Geometry: final body of the model. Coordinates: model frame, mm. A direction names the side the tool comes from. Give positions to 0.01 mm unless a question says otherwise; leave off trailing zeros. Order: outer loops, then holes, each group sorted by start corner. A loop starts at its lowest first (then second) coordinate and runs counter-clockwise, first axis right, second up. Notation, with made-up numbers: (-3.5, 66.25) - (35.5, 66.25) arc R31 cw to (35.5, 90.25) - close; hole circle Ø8 at (10, 89.25). An arc over 180 degrees is marked (long way). Use one line per item in the form item = value.
from build123d import *

# Parameters (mm, degrees)
SKETCH1_W           = 117.5
SKETCH1_H           = 85
BOSS_EXTRUDE1_DEPTH = 3
SKETCH2_W           = 17.5
SKETCH2_H           = 5
BOSS_EXTRUDE2_DEPTH = 94
SKETCH3_W           = 17.5
SKETCH3_H           = 20
SKETCH3_R           = 2.1
BOSS_EXTRUDE3_DEPTH = 5
CHAMFER1_SIZE       = 2
CHAMFER2_SIZE       = 3
FILLET1_R           = 4.2


with BuildPart() as part:
    # Sketch1 → Boss-Extrude1 (new body)
    with BuildSketch(Plane(origin=(0, 0, 0), x_dir=(1, 0, 0), z_dir=(0, 1, 0))):
        Rectangle(SKETCH1_W, SKETCH1_H)
    extrude(amount=BOSS_EXTRUDE1_DEPTH)

    # Sketch2 → Boss-Extrude2 (add)
    with BuildSketch(Plane(origin=(0, 3, 0), x_dir=(1, 0, 0), z_dir=(0, 1, 0))):
        with Locations((-50, 40)):
            Rectangle(SKETCH2_W, SKETCH2_H)
        with Locations((50, 40)):
            Rectangle(SKETCH2_W, SKETCH2_H)
        with Locations((50, -40)):
            Rectangle(SKETCH2_W, SKETCH2_H)
        with Locations((-50, -40)):
            Rectangle(SKETCH2_W, SKETCH2_H)
    extrude(amount=BOSS_EXTRUDE2_DEPTH)

    # Sketch3 → Boss-Extrude3 (add)
    # profile 1 of 4: a face of its own
    with BuildSketch(Plane(origin=(0, 97, 0), x_dir=(1, 0, 0), z_dir=(0, 1, 0))):
        with Locations((-50, 47.5)):
            Rectangle(SKETCH3_W, SKETCH3_H)
        with Locations(Location((-50, 50, 0), (0, 0, 270))):
            Circle(SKETCH3_R, mode=Mode.SUBTRACT)
    # profile 2 of 4: a face of its own
    with BuildSketch(Plane(origin=(0, 97, 0), x_dir=(1, 0, 0), z_dir=(0, 1, 0))):
        with Locations((50, 47.5)):
            Rectangle(SKETCH3_W, SKETCH3_H)
        with Locations(Location((50, 50, 0), (0, 0, 90))):
            Circle(SKETCH3_R, mode=Mode.SUBTRACT)
    # profile 3 of 4: a face of its own
    with BuildSketch(Plane(origin=(0, 97, 0), x_dir=(1, 0, 0), z_dir=(0, 1, 0))):
        with Locations((50, -47.5)):
            Rectangle(SKETCH3_W, SKETCH3_H)
        with Locations(Location((50, -50, 0), (0, 0, 270))):
            Circle(SKETCH3_R, mode=Mode.SUBTRACT)
    # profile 4 of 4: a face of its own
    with BuildSketch(Plane(origin=(0, 97, 0), x_dir=(1, 0, 0), z_dir=(0, 1, 0))):
        with Locations((-50, -47.5)):
            Rectangle(SKETCH3_W, SKETCH3_H)
        with Locations(Location((-50, -50, 0), (0, 0, 90))):
            Circle(SKETCH3_R, mode=Mode.SUBTRACT)
    extrude(amount=-BOSS_EXTRUDE3_DEPTH)

    # Chamfer1
    chamfer1_edges = [part.edges().sort_by_distance(p)[0] for p in [
        (50, 92, 47.9),
        (-50, 92, 52.1),
        (-50, 92, -52.1),
        (50, 92, -47.9),
    ]]
    chamfer(chamfer1_edges, length=CHAMFER1_SIZE)

    # Chamfer2
    chamfer2_edges = [part.edges().sort_by_distance(p)[0] for p in [
        (50, 92, 42.5),
        (-50, 92, 42.5),
        (-50, 92, -42.5),
        (50, 92, -42.5),
    ]]
    chamfer(chamfer2_edges, length=CHAMFER2_SIZE)

    # Fillet1
    fillet1_edges = [part.edges().sort_by_distance(p)[0] for p in [
        (41.25, 94.5, 57.5),
        (58.75, 94.5, 57.5),
        (-58.75, 94.5, 57.5),
        (-41.25, 94.5, 57.5),
        (-41.25, 94.5, -57.5),
        (-58.75, 94.5, -57.5),
        (58.75, 94.5, -57.5),
        (41.25, 94.5, -57.5),
    ]]
    fillet(fillet1_edges, radius=FILLET1_R)


solid = part.part
(1) Cut plane D-D on z = -39.5. Output: boundary loops of the cut face in (x, y).
Computed values:
outline = (-58.75, 0) - (58.75, 0) - (58.75, 97) - (41.25, 97) - (41.25, 3) - (-41.25, 3) - (-41.25, 97) - (-58.75, 97) - close
(2) Cut plane C-C on z = 50. Output: boundary loops of the cut face in (x, y), plus the area to 3 significant figures.
Computed values:
outline = (-58.75, 92) - (-54.1, 92) - (-52.1, 94) - (-52.1, 97) - (-58.75, 97) - close; (-47.9, 94) - (-45.9, 92) - (-41.25, 92) - (-41.25, 97) - (-47.9, 97) - close; (41.25, 92) - (45.9, 92) - (47.9, 94) - (47.9, 97) - (41.25, 97) - close; (52.1, 94) - (54.1, 92) - (58.75, 92) - (58.75, 97) - (52.1, 97) - close
area = 125 mm²
(3) Cut plane B-B on x = -50. Output: boundary loops of the cut face in (y, z).
Computed values:
outline = (0, -42.5) - (89, -42.5) - (92, -45.5) - (92, -45.9) - (94, -47.9) - (97, -47.9) - (97, -37.5) - (3, -37.5) - (3, 37.5) - (97, 37.5) - (97, 47.9) - (94, 47.9) - (92, 45.9) - (92, 45.5) - (89, 42.5) - (0, 42.5) - close; (92, -57.5) - (97, -57.5) - (97, -52.1) - (94, -52.1) - (92, -54.1) - close; (92, 54.1) - (94, 52.1) - (97, 52.1) - (97, 57.5) - (92, 57.5) - close
(4) Ray query, line 1 along X through (y, z) = (95.7, 50); line 2 along Z through (x, y) = (-43, 45); line 3 along Y through (x, z) = (23.5, -32). Return the intervals inside material, ascending.
Computed values:
line_1 = -58.75 to -52.1, -47.9 to -41.25, 41.25 to 47.9, 52.1 to 58.75
line_2 = -42.5 to -37.5, 37.5 to 42.5
line_3 = 0 to 3
(5) Pull-direction query (X, two-part tool) for faces 1 (the face through (58.75, 41, 40)), 2 (the face through (-48.137, 95.521, 49.031)), 3 (the face through (50, 95, 57.5)), 4 (the face through (42.45, 94.46, 56.24)); classes: released by +X, released by -X, zero draft, split by the parting line, or undercut.
Computed values:
face_1 = released by +X
face_2 = undercut
face_3 = zero draft
face_4 = undercut
(6) Cut plane A-A on y = 24.5. Output: boundary loops of the cut face in (x, z).
Computed values:
outline = (-58.75, -42.5) - (-41.25, -42.5) - (-41.25, -37.5) - (-58.75, -37.5) - close; (-58.75, 37.5) - (-41.25, 37.5) - (-41.25, 42.5) - (-58.75, 42.5) - close; (41.25, -42.5) - (58.75, -42.5) - (58.75, -37.5) - (41.25, -37.5) - close; (41.25, 37.5) - (58.75, 37.5) - (58.75, 42.5) - (41.25, 42.5) - close
(7) Contact query for flat-ended pins moving along their axis: pin 1 Ø9.5 at (x, z) = (-46, 51.5) entering from -Y; pin 2 Ø3.5 at (x, z) = (-50, -50) entering from +Y; pin 3 Ø9.5 at (x, z) = (-51.5, -48.5) entering from -Y; pin 4 Ø5 at (x, y) = (-47, 65.5) entering from +Z. Output: stop coordinate, or through.
Computed values:
pin_1 = 92
pin_2 = through
pin_3 = 90.25
pin_4 = 42.5
(8) Reachability of faces 5 (the face through (4, 1, 42.5)), 6 (the face through (49.9, 97, -47.6)), 7 (the face through (-41.25, 53, -42)), 8 (the face through (-50, 49, -37.5)) from +Z, -Z, +X, -X, +Y, -Y: full face, straight path, thin tool, end or side. Return the list, or none.
Computed values:
face_5 = +Z, +X, -X, -Y
face_6 = +Z, -Z, +X, -X, +Y
face_7 = +Z, -Z, +Y
face_8 = +X, -X, +Y
